from build123d import *

# Parameters (mm, degrees)
BOX010_W               = 11
BOX010_H               = 3
BOX010_DEPTH           = 3
BOX010_PLACEMENT_ANGLE = 60.000023
BOX004_W               = 26
BOX004_H               = 10
BOX004_DEPTH           = 10
BOX005_W               = 8
BOX005_H               = 10
BOX005_DEPTH           = 13
BOX006_W               = 10
BOX006_H               = 13.6
BOX006_DEPTH           = 9.7
BOX007_W               = 6
BOX007_H               = 13.6
BOX007_DEPTH           = 8.2
BOX008_W               = 8
BOX008_H               = 10
BOX008_DEPTH           = 10
BOX009_W               = 11
BOX009_H               = 3
BOX009_DEPTH           = 3
BOX009_PLACEMENT_ANGLE = 29.99999
CYLINDER012024_R       = 1.85
CYLINDER012024_DEPTH   = 15.8
CYLINDER012026_R       = 5.5
CYLINDER012026_DEPTH   = 17.5
BOX003_W               = 5
BOX003_H               = 17.5
BOX003_DEPTH           = 4
BOX001_W               = 7
BOX001_H               = 18
BOX001_DEPTH           = 4
CYLINDER012025_R       = 6.85
CYLINDER012025_DEPTH   = 3
CYLINDER012023_R       = 2.45
CYLINDER012023_DEPTH   = 17.5
CYLINDER012022_R       = 6.85
CYLINDER012022_DEPTH   = 3
BOX002_W               = 9
BOX002_H               = 18
BOX002_DEPTH           = 5
BOX002_PLACEMENT_ANGLE = 35.00002
BOX_W                  = 24
BOX_H                  = 16.6
BOX_DEPTH              = 13
FILLET_R               = 6.4


with BuildPart() as box010:
    # Box010 → Box010 (new body)
    with BuildSketch(Plane.XY):
        with Locations((5.5, 1.5)):
            Rectangle(BOX010_W, BOX010_H)
    extrude(amount=BOX010_DEPTH)


with BuildPart() as box010_1:
    # Box010 placement: moved
    add(box010.part.moved(Location((12.5, 13.7, 7.1))).rotate(Axis((12.5, 13.7, 7.1), (1, 0, 0)), BOX010_PLACEMENT_ANGLE))


with BuildPart() as box004:
    # Box004 → Box004 (new body)
    with BuildSketch(Plane(origin=(-1, 3.4, 1.5), x_dir=(1, 0, 0), z_dir=(0, 0, 1))):
        with Locations((13, 5)):
            Rectangle(BOX004_W, BOX004_H)
    extrude(amount=BOX004_DEPTH)


with BuildPart() as box005:
    # Box005 → Box005 (new body)
    with BuildSketch(Plane(origin=(-1, 3.4, -1.5), x_dir=(1, 0, 0), z_dir=(0, 0, 1))):
        with Locations((4, 5)):
            Rectangle(BOX005_W, BOX005_H)
    extrude(amount=BOX005_DEPTH)


with BuildPart() as box006:
    # Box006 → Box006 (new body)
    with BuildSketch(Plane(origin=(15.35, 1.6, 0), x_dir=(1, 0, 0), z_dir=(0, 0, 1))):
        with Locations((5, 6.8)):
            Rectangle(BOX006_W, BOX006_H)
    extrude(amount=BOX006_DEPTH)


with BuildPart() as box007:
    # Box007 → Box007 (new body)
    with BuildSketch(Plane(origin=(12.5, 1.6, 1.5), x_dir=(1, 0, 0), z_dir=(0, 0, 1))):
        with Locations((3, 6.8)):
            Rectangle(BOX007_W, BOX007_H)
    extrude(amount=BOX007_DEPTH)


with BuildPart() as box008:
    # Box008 → Box008 (new body)
    with BuildSketch(Plane(origin=(15.35, 3.4, 3.5), x_dir=(1, 0, 0), z_dir=(0, 0, 1))):
        with Locations((4, 5)):
            Rectangle(BOX008_W, BOX008_H)
    extrude(amount=BOX008_DEPTH)


with BuildPart() as fusion011:
    # Box009 → Box009 (new body)
    with BuildSketch(Plane.XY):
        with Locations((5.5, 1.5)):
            Rectangle(BOX009_W, BOX009_H)
    extrude(amount=BOX009_DEPTH)


with BuildPart() as fusion011_1:
    # Box009 placement: moved
    add(fusion011.part.moved(Location((12.5, 3.1, 7.1))).rotate(Axis((12.5, 3.1, 7.1), (1, 0, 0)), BOX009_PLACEMENT_ANGLE))

    # Fusion011: union Box010, Box004, Box005, Box006, Box007, Box008
    add(box010_1.part)
    add(box004.part)
    add(box005.part)
    add(box006.part)
    add(box007.part)
    add(box008.part)


with BuildPart() as cylinder012024:
    # Cylinder012024 → Cylinder012024 (new body)
    with BuildSketch(Plane(origin=(4.5, 16.3, 6.5), x_dir=(1, 0, 0), z_dir=(0, -1, 0))):
        Circle(CYLINDER012024_R)
    extrude(amount=CYLINDER012024_DEPTH)


with BuildPart() as cylinder012026:
    # Cylinder012026 → Cylinder012026 (new body)
    with BuildSketch(Plane(origin=(5, 17, 5.5), x_dir=(1, 0, 0), z_dir=(0, -1, 0))):
        Circle(CYLINDER012026_R)
    extrude(amount=CYLINDER012026_DEPTH)


with BuildPart() as cut003004:
    # Box003 → Box003 (new body)
    with BuildSketch(Plane(origin=(0, -0.5, 0), x_dir=(1, 0, 0), z_dir=(0, 0, 1))):
        with Locations((2.5, 8.75)):
            Rectangle(BOX003_W, BOX003_H)
    extrude(amount=BOX003_DEPTH)

    # Cut003004: cut Cylinder012026
    add(cylinder012026.part, mode=Mode.SUBTRACT)


with BuildPart() as box001:
    # Box001 → Box001 (new body)
    with BuildSketch(Plane(origin=(3.2, -1, 9.9), x_dir=(1, 0, 0), z_dir=(0, 0, 1))):
        with Locations((3.5, 9)):
            Rectangle(BOX001_W, BOX001_H)
    extrude(amount=BOX001_DEPTH)


with BuildPart() as cylinder012025:
    # Cylinder012025 → Cylinder012025 (new body)
    with BuildSketch(Plane(origin=(4.6, 2, 6.5), x_dir=(1, 0, 0), z_dir=(0, -1, 0))):
        Circle(CYLINDER012025_R)
    extrude(amount=CYLINDER012025_DEPTH)


with BuildPart() as cylinder012023:
    # Cylinder012023 → Cylinder012023 (new body)
    with BuildSketch(Plane(origin=(19, 17, 6.5), x_dir=(1, 0, 0), z_dir=(0, -1, 0))):
        Circle(CYLINDER012023_R)
    extrude(amount=CYLINDER012023_DEPTH)


with BuildPart() as cylinder012022:
    # Cylinder012022 → Cylinder012022 (new body)
    with BuildSketch(Plane(origin=(4.6, 17.8, 6.5), x_dir=(1, 0, 0), z_dir=(0, -1, 0))):
        Circle(CYLINDER012022_R)
    extrude(amount=CYLINDER012022_DEPTH)


with BuildPart() as fusion012:
    # Box002 → Box002 (new body)
    with BuildSketch(Plane.XY):
        with Locations((4.5, 9)):
            Rectangle(BOX002_W, BOX002_H)
    extrude(amount=BOX002_DEPTH)


with BuildPart() as fusion012_1:
    # Box002 placement: moved
    add(fusion012.part.moved(Location((-0.8, -1, 6.4))).rotate(Axis((-0.8, -1, 6.4), (0, -1, 0)), BOX002_PLACEMENT_ANGLE))

    # Fusion010: union Box001, Cylinder012025, Cylinder012023, Cylinder012022
    add(box001.part)
    add(cylinder012025.part)
    add(cylinder012023.part)
    add(cylinder012022.part)

    # Fusion012: union Cut003004
    add(cut003004.part)


with BuildPart() as pieza:
    # Box → Box (new body)
    with BuildSketch(Plane(origin=(0, 0.1, 0), x_dir=(1, 0, 0), z_dir=(0, 0, 1))):
        with Locations((12, 8.3)):
            Rectangle(BOX_W, BOX_H)
    extrude(amount=BOX_DEPTH)

    # Fillet
    fillet_edges = [pieza.edges().sort_by_distance(p)[0] for p in [
        (24, 8.4, 13),
        (24, 8.4, 0),
    ]]
    fillet(fillet_edges, radius=FILLET_R)

    # Cut003005: cut Fusion012
    add(fusion012_1.part, mode=Mode.SUBTRACT)

    # Fusion013: union Cylinder012024
    add(cylinder012024.part)

    # Cut002007: cut Fusion011
    add(fusion011_1.part, mode=Mode.SUBTRACT)


with BuildPart() as pieza_1:
    # Cut002007 placement: moved
    add(pieza.part.moved(Location((-4.5, -8, -6.5))))


solid = pieza_1.part
The model under review builds one solid part; all positions refer to its coordinate system, in mm. A direction names the side the tool comes from. Coordinates: 2 decimals unless noted, no trailing zeros. Write each loop counter-clockwise with the first axis right and the second up, starting at its lowest first coordinate (ties: lowest second). Pieces come first, ordered by that corner, then holes. Notation, with made-up numbers: M 37,85 L 79,85 A24 ccw 79,106 Z; hole C 29.25,-33.75 d4. An arc over 180 degrees is marked long. Put each result on its own line as item: value.
1) Clearance check with flat-ended pins moving along their axes: pin 1 Ø1 at (x, y) = (14, 5.5) entering from -Z; pin 2 Ø1.4 at (y, z) = (-5, 0.5) entering from +X; pin 3 Ø1.5 at (y, z) = (1, 4) entering from +X; pin 4 Ø0.8 at (y, z) = (3, -6) entering from +X. State where each tip first meets the part, or that it passes through.
Computed:
pin 1: stops at z = 3.89
pin 2: stops at x = 8
pin 3: passes through
pin 4: stops at x = 10.85
2) Draft analysis for pull direction X (two halves, no side actions). For faces 1 (the flat face through (5.7, 0.3, 5.3)), 2 (the flat face through (4, 5.4, 0)), 3 (the cylindrical face through (6.578, -6.937, -2.227)), state which applies: released by +X, released by -X, zero draft, split by the parting line, or undercut.
Computed:
face 1: released by -X
face 2: zero draft
face 3: undercut
3) For faces 4 (the cylindrical face through (6.578, 7.763, -2.227)), 5 (the flat face through (8, 0, 5)), 6 (the flat face through (12, 7.2, -2)), 7 (the flat face through (3, 6, 3.4)), 8 (the flat face through (1, -6, -2)), list the 3-axis set-ups (+Z, -Z, +X, -X, +Y, -Y) from which the entire face can be reached by the end or side of a thin tool; tool diameter is ignored.
Computed:
face 4: +Y
face 5: +X, -X
face 6: +X
face 7: +Z, -X, +Y, -Y
face 8: -Y
4) Add section A-A on y = -3. Give the boundary of the cut face in (x, z).
Computed:
outline: M 2.5,-6.5 L 10.85,-6.5 L 10.85,-5 L 2.5,-5 Z; M 5.7,5 L 10.85,5 L 10.85,6.5 L 5.7,6.5 Z
5) Add section D-D on x = 14.5. State how many separate pieces and enclosed holes the cut face has, then the cut area to 3 significant figures.
Computed:
separate pieces: 4
enclosed holes: 0
area: 32.8 mm2
6) Add section B-B on x = -3. Give the boundary of the cut face in (y, z).
Computed:
outline: M -6,-5.24 L -4.6,-5.24 L -4.6,1.51 L -6,1.51 Z; M 5.4,-5.24 L 6.8,-5.24 L 6.8,1.51 L 5.4,1.51 Z
7) Add section C-C on z = -4. Give the boundary of the cut face in (x, y).
Computed:
outline: M -4.11,-6 L 5.66,-6 L 5.66,-7.9 L 18.17,-7.9 L 18.17,-6.4 L 8,-6.4 L 8,-4.6 L -4.11,-4.6 Z; M -4.11,5.4 L 8,5.4 L 8,7.2 L 18.17,7.2 L 18.17,8.7 L 5.66,8.7 L 5.66,6.8 L -4.11,6.8 Z
8) Wall thickness on probe 1 along X at (y, z) = (-6.7, 0); probe 2 along Y at (x, z) = (-2.5, -4); probe 3 along Y at (x, z) = (9.5, -2.75): over which ranges is each line inside the solid? List them lowest first. Write a range as [from, to].
Computed:
probe 1: x = [-1.85, 1.85], [6.95, 12.05], [16.95, 19.5]
probe 2: y = [-6, -4.6], [5.4, 6.8]
probe 3: y = [-7.9, -6.4], [7.2, 8.7]
